Model file for the job. Use its own axes, mm. A direction names the side the tool comes from. Round coordinates to 2 decimals unless told otherwise and drop trailing zeros. Loops run counter-clockwise (first coordinate to the right, second up) from the corner with the lowest first, then second, coordinate; pieces in that order, holes last. Notation, with made-up numbers: (-26.75, -34) - (10.25, -34) arc R21 ccw to (10.25, -2) - close; hole circle Ø11 at (-12, -9.5). An arc over 180 degrees is marked (long way). Use one line per item in the form item = value.
from build123d import *

# Parameters (mm, degrees)
BOSS_EXTRUDE1_DEPTH = 4
SKETCH2_R           = 2
CUT_EXTRUDE1_DEPTH  = 4
SKETCH3_R           = 5
CUT_EXTRUDE2_DEPTH  = 2
SKETCH4_R           = 40
SKETCH4_R_2         = 36
BOSS_EXTRUDE2_DEPTH = 70


with BuildPart() as part:
    # Sketch1 → Boss-Extrude1 (new body)
    with BuildSketch(Plane(origin=(0, 0, 0), x_dir=(1, 0, 0), z_dir=(0, 1, 0))):
        with BuildLine():
            Line((-47.5, 7.5), (-34.114378278, 20.885621722))
            ThreePointArc((-34.114378278, 20.885621722), (-28.284271247, 28.284271247), (-20.885621722, 34.114378278))
            Line((-20.885621722, 34.114378278), (-7.5, 47.5))
            ThreePointArc((-7.5, 47.5), (0, 55), (7.5, 47.5))
            Line((7.5, 47.5), (20.885621722, 34.114378278))
            ThreePointArc((20.885621722, 34.114378278), (28.284271247, 28.284271247), (34.114378278, 20.885621722))
            Line((34.114378278, 20.885621722), (47.5, 7.5))
            ThreePointArc((47.5, 7.5), (55, 0), (47.5, -7.5))
            Line((47.5, -7.5), (34.114378278, -20.885621722))
            ThreePointArc((34.114378278, -20.885621722), (28.284271247, -28.284271247), (20.885621722, -34.114378278))
            Line((20.885621722, -34.114378278), (7.5, -47.5))
            ThreePointArc((7.5, -47.5), (0, -55), (-7.5, -47.5))
            Line((-7.5, -47.5), (-20.885621722, -34.114378278))
            ThreePointArc((-20.885621722, -34.114378278), (-28.284271247, -28.284271247), (-34.114378278, -20.885621722))
            Line((-34.114378278, -20.885621722), (-47.5, -7.5))
            ThreePointArc((-47.5, -7.5), (-55, 0), (-47.5, 7.5))
        make_face()
    extrude(amount=BOSS_EXTRUDE1_DEPTH)

    # Sketch2 → Cut-Extrude1 (cut)
    with BuildSketch(Plane(origin=(0, 4, 0), x_dir=(1, 0, 0), z_dir=(0, 1, 0))):
        with Locations(Location((-47.5, 0, 0), (0, 0, 270))):
            Circle(SKETCH2_R)
        with Locations(Location((0, 47.5, 0), (0, 0, 270))):
            Circle(SKETCH2_R)
        with Locations(Location((47.5, 0, 0), (0, 0, 270))):
            Circle(SKETCH2_R)
        with Locations(Location((0, -47.5, 0), (0, 0, 270))):
            Circle(SKETCH2_R)
    extrude(amount=-CUT_EXTRUDE1_DEPTH, mode=Mode.SUBTRACT)

    # Sketch3 → Cut-Extrude2 (cut)
    with BuildSketch(Plane(origin=(0, 4, 0), x_dir=(1, 0, 0), z_dir=(0, 1, 0))):
        with Locations(Location((-47.5, 0, 0), (0, 0, 270))):
            Circle(SKETCH3_R)
        with Locations(Location((0, 47.5, 0), (0, 0, 270))):
            Circle(SKETCH3_R)
        with Locations(Location((47.5, 0, 0), (0, 0, 270))):
            Circle(SKETCH3_R)
        with Locations(Location((0, -47.5, 0), (0, 0, 270))):
            Circle(SKETCH3_R)
    extrude(amount=-CUT_EXTRUDE2_DEPTH, mode=Mode.SUBTRACT)

    # Sketch4 → Boss-Extrude2 (add)
    with BuildSketch(Plane(origin=(0, 4, 0), x_dir=(1, 0, 0), z_dir=(0, 1, 0))):
        with Locations(Location((0, 0, 0), (0, 0, 58.524055273))):
            Circle(SKETCH4_R)
        with Locations(Location((0, 0, 0), (0, 0, 270))):
            Circle(SKETCH4_R_2, mode=Mode.SUBTRACT)
    extrude(amount=BOSS_EXTRUDE2_DEPTH)


solid = part.part
1. Tool access for faces 4 (the flat face through (0, 4, -42)), 5 (the cylindrical face through (0.22, 3.014, 42.505)), 6 (the flat face through (-41, 2, -14)): list every direction of +Z, -Z, +X, -X, +Y, -Y with a clear straight run to the whole face (end or side of a thin tool).
Geometry check:
face_4 = -Z, +Y
face_5 = +Y
face_6 = -Z, -X, +Y, -Y
2. Pull direction X, two halves, no side cores. Call faces 1 (the flat face through (1, 0, -1)), 2 (the cylindrical face through (0, 2, -55)), 3 (the cylindrical face through (52.457, 3.014, -0.651)): +X half, -X half, draft (parallel to the pull), parting line (faces both ways), or undercut.
Geometry check:
face_1 = draft
face_2 = parting line
face_3 = undercut
3. Cut at C-C, the plane y = 26. Give the cut face in (x, z), plus the area to 3 significant figures.
Geometry check:
outline = circle Ø80 at (0, 0); hole circle Ø72 at (0, 0)
area = 955 mm^2
4. Wall check: probe 1 along X at (y, z) = (0.7, 0); probe 2 along X at (y, z) = (2.6, 47.5); probe 3 along X at (y, z) = (3, 0). Give the ranges that are in metal, low to high.
Geometry check:
probe_1 = -55 to -49.5, -45.5 to 45.5, 49.5 to 55
probe_2 = -7.5 to -5, 5 to 7.5
probe_3 = -55 to -52.5, -42.5 to 42.5, 52.5 to 55
5. Cut at B-B, the plane z = -32. Give the cut face in (x, y), plus the area to 3 significant figures.
Geometry check:
outline = (-24, 0) - (24, 0) - (24, 74) - (16.49, 74) - (16.49, 4) - (-16.49, 4) - (-16.49, 74) - (-24, 74) - close
area = 1,240 mm^2
6. Flat gauge pins, fed straight in: pin 1 (11 mm diameter, centred on x = -49, z = 2, fed in from +Y); pin 2 (2 mm diameter, centred on y = 22, z = -11.5, fed in from +X); pin 3 (6 mm diameter, centred on x = 33, y = 35.5, fed in from -Z). Where does each tip first touch, or does it go through?
Geometry check:
pin_1 = 4
pin_2 = 38.6
pin_3 = -26.46
7. Cut at A-A, the plane x = 0. Give the cut face in (y, z).
Geometry check:
outline = (0, -55) - (4, -55) - (4, -52.5) - (2, -52.5) - (2, -49.5) - (0, -49.5) - close; (0, -45.5) - (2, -45.5) - (2, -42.5) - (4, -42.5) - (4, -40) - (74, -40) - (74, -36) - (4, -36) - (4, 36) - (74, 36) - (74, 40) - (4, 40) - (4, 42.5) - (2, 42.5) - (2, 45.5) - (0, 45.5) - close; (0, 49.5) - (2, 49.5) - (2, 52.5) - (4, 52.5) - (4, 55) - (0, 55) - close
8. Cut at D-D, the plane x = -16. Give the cut face in (y, z).
Geometry check:
outline = (0, -39) - (4, -39) - (4, -36.66) - (74, -36.66) - (74, -32.25) - (4, -32.25) - (4, 32.25) - (74, 32.25) - (74, 36.66) - (4, 36.66) - (4, 39) - (0, 39) - close
